from build123d import *

# Parameters (mm, degrees)
SZKIC1_R                    = 1.63
SZKIC1_R_2                  = 1.627886045
SZKIC1_R_3                  = 1.634186666
SZKIC1_R_4                  = 1.631321013
DODANIE_WYCI_GNI_CIE1_DEPTH = 37.7
SZKIC2_W                    = 96.882996132
SZKIC2_H                    = 10
WYTNIJ_WYCI_GNI_CIE1_DEPTH  = 3.027599165
SZKIC4_W                    = 27.7
SZKIC4_H                    = 3.027599165
DODANIE_WYCI_GNI_CIE2_DEPTH = 4.6
SZKIC5_W                    = 27.7
SZKIC5_H                    = 3.027593756
DODANIE_WYCI_GNI_CIE4_DEPTH = 4.6
WYTNIJ_WYCI_GNI_CIE2_REACH  = 74.407
SZKIC6_R                    = 2.5
SZKIC7_W                    = 110.003784397
SZKIC7_H                    = 59.74457964
WYTNIJ_WYCI_GNI_CIE4_DEPTH  = 30.7


with BuildPart() as part:
    # Szkic1 → Dodanie-wyciągnięcie1 (new body)
    with BuildSketch(Plane(origin=(0, 0, 0), x_dir=(-1, 0, 0), z_dir=(0, 0, 1))):
        with BuildLine():
            Line((-42.206476447, -1.143440143), (-42.187291437, -4.170973113))
            Line((-42.187291437, -4.170973113), (54.693759689, -3.557073712))
            Line((54.693759689, -3.557073712), (54.674575297, -0.529535329))
            Line((54.674575297, -0.529535329), (31.895047363, -0.673880775))
            ThreePointArc((31.895047363, -0.673880775), (30.123615765, 0.046208772), (29.379274421, 1.807587444))
            Line((29.379274421, 1.807587444), (29.351860706, 5.515732081))
            ThreePointArc((29.351860706, 5.515732081), (27.236675167, 10.484490063), (22.240808109, 12.534826154))
            Line((22.240808109, 12.534826154), (20.472861468, 12.523590896))
            ThreePointArc((20.472861468, 12.523590896), (19.415024557, 12.077529638), (18.982423849, 11.01411711))
            Line((18.982423849, 11.01411711), (18.989158593, 9.951213651))
            ThreePointArc((18.989158593, 9.951213651), (19.04575769, 9.79437408), (19.188385802, 9.708006664))
            Line((19.188385802, 9.708006664), (22.37305409, 9.047530924))
            Line((22.37305409, 9.047530924), (22.37305409, 7.841359432))
            Line((22.37305409, 7.841359432), (14.677855674, 7.841359432))
            ThreePointArc((14.677855674, 7.841359432), (4.517774256, 5.390280076), (-5.642307162, 7.841359432))
            Line((-5.642307162, 7.841359432), (-11.13863745, 7.841359432))
            ThreePointArc((-11.13863745, 7.841359432), (-11.344351569, 7.733421748), (-11.372431243, 7.502813045))
            Line((-11.372431243, 7.502813045), (-9.580573211, 2.77167383))
            Line((-9.580573211, 2.77167383), (-9.53660226, 2.594556029))
            ThreePointArc((-9.53660226, 2.594556029), (-10.047085724, 1.71578131), (-10.990723107, 2.09312315))
            Line((-10.990723107, 2.09312315), (-11.062286258, 2.28207519))
            Line((-11.062286258, 2.28207519), (-13.125087597, 7.728600603))
            ThreePointArc((-13.125087597, 7.728600603), (-13.0127689, 8.651035416), (-12.189912428, 9.082786152))
            Line((-12.189912428, 9.082786152), (-11.351176976, 9.082786152))
            ThreePointArc((-11.351176976, 9.082786152), (-11.174400281, 9.156009457), (-11.101176976, 9.332786152))
            Line((-11.101176976, 9.332786152), (-11.101176976, 9.341072815))
            ThreePointArc((-11.101176976, 9.341072815), (-11.158575506, 9.873705952), (-11.328135423, 10.381881202))
            Line((-11.328135423, 10.381881202), (-11.52139656, 10.803947934))
            ThreePointArc((-11.52139656, 10.803947934), (-11.948131465, 11.44871119), (-12.551468508, 11.932246866))
            Line((-12.551468508, 11.932246866), (-15.002316135, 13.336662904))
            ThreePointArc((-15.002316135, 13.336662904), (-15.916443983, 13.645833839), (-16.879567484, 13.585754641))
            Line((-16.879567484, 13.585754641), (-17.376357402, 13.455449083))
            ThreePointArc((-17.376357402, 13.455449083), (-19.591854135, 11.040960081), (-18.31207326, 8.024282466))
            Line((-18.31207326, 8.024282466), (-15.235252345, 4.594263276))
            ThreePointArc((-15.235252345, 4.594263276), (-14.894447251, 2.450948387), (-16.707962408, 1.258845372))
            Line((-16.707962408, 1.258845372), (-16.931951142, 1.257044798))
            ThreePointArc((-16.931951142, 1.257044798), (-17.929768207, 0.793667315), (-18.054097125, -0.299447458))
            ThreePointArc((-18.054097125, -0.299447458), (-18.09762478, -0.768632421), (-18.511820167, -0.993290758))
            Line((-18.511820167, -0.993290758), (-42.206476447, -1.143440143))
        make_face()
        with Locations(Location((21.198480742, 2.425447379, 0), (0, 0, 180))):
            Circle(SZKIC1_R, mode=Mode.SUBTRACT)
        with Locations(Location((-4.937145948, 2.427386246, 0), (0, 0, 180))):
            Circle(SZKIC1_R_2, mode=Mode.SUBTRACT)
        with Locations(Location((3.802928012, 2.422545785, 0), (0, 0, 180))):
            Circle(SZKIC1_R_3, mode=Mode.SUBTRACT)
        with Locations(Location((12.538480742, 2.425447379, 0), (0, 0, 180))):
            Circle(SZKIC1_R_4, mode=Mode.SUBTRACT)
    extrude(amount=DODANIE_WYCI_GNI_CIE1_DEPTH)

    # Szkic2 → Wytnij-wyciągnięcie1 (cut)
    with BuildSketch(Plane(origin=(-0.02473498, 3.903491109, 0), x_dir=(0.9999799241630359, 0.006336503048932176, 0), z_dir=(-0.006336503048932176, 0.9999799241630359, 0))):
        with Locations((-6.228624191, -32.7)):
            Rectangle(SZKIC2_W, SZKIC2_H)
    extrude(amount=-WYTNIJ_WYCI_GNI_CIE1_DEPTH, mode=Mode.SUBTRACT)

    # Szkic4 → Dodanie-wyciągnięcie2 (add)
    with BuildSketch(Plane(origin=(-54.669024709, -0.346417396, 0), x_dir=(0, 0, 1), z_dir=(-0.9999799241630359, -0.006336503048932243, 0))):
        with Locations((13.85, 2.389769894)):
            Rectangle(SZKIC4_W, SZKIC4_H)
    extrude(amount=DODANIE_WYCI_GNI_CIE2_DEPTH)

    # Szkic5 → Dodanie-wyciągnięcie4 (add)
    with BuildSketch(Plane(origin=(42.212027201, 0.26749111, 0), x_dir=(0, 0, -1), z_dir=(0.9999799227968423, 0.00633671864778665, 0))):
        with Locations((-13.85, 2.389763497)):
            Rectangle(SZKIC5_W, SZKIC5_H)
    extrude(amount=DODANIE_WYCI_GNI_CIE4_DEPTH)

    # Wytnij-wyciągnięcie2: up to this face of the body (flat: up to its plane)
    wytnij_wyci_gni_cie2_end = Plane(part.part.faces().sort_by_distance((-45.584765156, 0.587134095, 13.85))[0])
    # Szkic6 → Wytnij-wyciągnięcie2 (cut, up to the picked face)
    with BuildSketch(Plane(origin=(-0.02473498, 3.903491109, 0), x_dir=(0.9999799241630359, 0.006336503048932172, 0), z_dir=(-0.006336503048932172, 0.9999799241630359, 0)), mode=Mode.PRIVATE) as wytnij_wyci_gni_cie2_sk1:
        with Locations((-53.770122257, -7.5)):
            Circle(SZKIC6_R)
    wytnij_wyci_gni_cie2_tool1 = split(extrude(wytnij_wyci_gni_cie2_sk1.sketch, amount=-WYTNIJ_WYCI_GNI_CIE2_REACH, mode=Mode.PRIVATE), bisect_by=wytnij_wyci_gni_cie2_end, keep=Keep.BOTH, mode=Mode.PRIVATE)
    # Szkic6 → Wytnij-wyciągnięcie2 (cut, up to the picked face)
    with BuildSketch(Plane(origin=(-0.02473498, 3.903491109, 0), x_dir=(0.9999799241630359, 0.006336503048932172, 0), z_dir=(-0.006336503048932172, 0.9999799241630359, 0)), mode=Mode.PRIVATE) as wytnij_wyci_gni_cie2_sk2:
        with Locations((41.312873875, -7.5)):
            Circle(SZKIC6_R)
    wytnij_wyci_gni_cie2_tool2 = split(extrude(wytnij_wyci_gni_cie2_sk2.sketch, amount=-WYTNIJ_WYCI_GNI_CIE2_REACH, mode=Mode.PRIVATE), bisect_by=wytnij_wyci_gni_cie2_end, keep=Keep.BOTH, mode=Mode.PRIVATE)
    add(wytnij_wyci_gni_cie2_tool1.solids().sort_by(Axis((-53.793778, 3.562777, 7.5), (0.006336503048932172, -0.9999799241630359, 0)))[0], mode=Mode.SUBTRACT)
    add(wytnij_wyci_gni_cie2_tool2.solids().sort_by(Axis((41.28731, 4.16527, 7.5), (0.006336503048932172, -0.9999799241630359, 0)))[0], mode=Mode.SUBTRACT)

    # Szkic7 → Wytnij-wyciągnięcie4 (cut)
    with BuildSketch(Plane(origin=(0, 0, 0), x_dir=(-1, 0, 0), z_dir=(0, 0, -1))):
        with Locations((7.955893791, -24.915165787)):
            Rectangle(SZKIC7_W, SZKIC7_H)
    extrude(amount=-WYTNIJ_WYCI_GNI_CIE4_DEPTH, mode=Mode.SUBTRACT)


with BuildPart() as wytnij_wyci_gni_cie4_kept_piece:
    # of the separate pieces the step leaves, the one the design keeps (wytnij_wyci_gni_cie4_pieces_kept)
    add(part.part.solids().sort_by_distance((18.31207326, -8.024282466, 30.7))[0])


solid = wytnij_wyci_gni_cie4_kept_piece.part
Check sheet for the modelled part. Datum: model origin and axes. Units: mm. A direction names the side the tool comes from. Give positions to 0.01 mm unless a question says otherwise; leave off trailing zeros. Write each loop counter-clockwise with the first axis right and the second up, starting at its lowest first coordinate (ties: lowest second). Pieces come first, ordered by that corner, then holes. Notation, with made-up numbers: (41, -36.5) -> (65, -36.5) arc R31 ccw to (65, -11.5) -> close; hole circle Ø10 at (-27.75, 80). An arc over 180 degrees is marked (long way). Use one line per item in the form item = value. Start each with the question number.
1. Section check A-A (x = 5). Record the cut outline in (y, z).
2. Go/stop test with flat-tipped pins: P1, Ø3, axis at x = -18.5, z = 34, coming from the +Y side; P2, Ø1.6, axis at x = 7.5, z = 35, coming from the -Y side; P3, Ø1.3, axis at y = -8, z = 32.5, coming from the +X side; P4, Ø2.5, axis at x = -12.54, y = -2.43, coming from the +Z side. Record where each tip stops, or that it passes through.
3. Section check B-B (y = -6.5). Record the cut outline in (x, z).
4. Mould release check, pull along Y, two halves, no side actions. Record for faces 5 (the cylindrical face through (17.92, -0.81, 34.15)), 6 (the flat face through (-6, -5, 30.7)), 7 (the flat face through (12, -9.083, 34)), 8 (the flat face through (13.76, -12.625, 34.151)): pulls with the +Y half, pulls with the -Y half, needs draft (parallel to the pull), parting line crosses it, or undercut.
5. Section check D-D (x = -12). Record the cut outline in (y, z).
6. Thickness scan on line 1 along X through (y, z) = (-7.75, 37); line 2 along X through (y, z) = (-7.25, 34.5); line 3 along X through (y, z) = (-2.5, 34). Record the ranges inside material, lowest first. Write a range as from..to.
7. Section check C-C (y = -3.5). Record the cut outline in (x, z), and give its area (3 significant figures).
8. Access from +Z, -Z, +X, -X, +Y, -Y to the whole of each face (thin tool, end or side, straight path). Record for faces 1 (the flat face through (-22.373, -8, 34)), 2 (the flat face through (16.795, -6.333, 34.151)), 3 (the flat face through (-6, -5, 37.7)), 4 (the cylindrical face through (11.157, -9.866, 34.151)).
Conclusion:
q1.outline = (-7.53, 30.7) -> (-4.05, 30.7) -> (-4.05, 37.7) -> (-7.53, 37.7) -> close; (-0.8, 30.7) -> (0.91, 30.7) -> (0.91, 37.7) -> (-0.8, 37.7) -> close
q2.P1 = 0.77
q2.P2 = -7.84
q2.P3 = 18.98
q2.P4 = through
q3.outline = (-29.27, 30.7) -> (-11.46, 30.7) -> (-11.46, 37.7) -> (-29.27, 37.7) -> close; (2.43, 30.7) -> (10.99, 30.7) -> (10.99, 37.7) -> (2.43, 37.7) -> close; (12.66, 30.7) -> (16.94, 30.7) -> (16.94, 37.7) -> (12.66, 37.7) -> close
q4.face_5 = undercut
q4.face_6 = needs draft
q4.face_7 = undercut
q4.face_8 = pulls with the -Y half
q5.outline = (-6.68, 30.7) -> (-3.97, 30.7) -> (-3.97, 37.7) -> (-6.68, 37.7) -> close; (-0.89, 30.7) -> (0.8, 30.7) -> (0.8, 37.7) -> (-0.89, 37.7) -> close
q6.line_1 = -28.96..-14.5, 5.46..11.33, 13.13..18.07
q6.line_2 = -29.11..-13.43, 4.39..11.28, 12.94..17.62
q6.line_3 = -29.37..-22.83, -19.57..-14.17, -10.91..-5.44, -2.17..3.31, 6.56..9.52, 11.14..14.87
q7.outline = (-29.37, 30.7) -> (-22.42, 30.7) -> (-22.42, 37.7) -> (-29.37, 37.7) -> close; (-19.97, 30.7) -> (-13.77, 30.7) -> (-13.77, 37.7) -> (-19.97, 37.7) -> close; (-11.31, 30.7) -> (-5.03, 30.7) -> (-5.03, 37.7) -> (-11.31, 37.7) -> close; (-2.57, 30.7) -> (3.71, 30.7) -> (3.71, 37.7) -> (-2.57, 37.7) -> close; (6.16, 30.7) -> (9.86, 30.7) -> (9.86, 37.7) -> (6.16, 37.7) -> close; (11.52, 30.7) -> (14.74, 30.7) -> (14.74, 37.7) -> (11.52, 37.7) -> close
q7.area = 228 mm²
q8.face_1 = +Z, -Z
q8.face_2 = +Z, -Z, +X
q8.face_3 = +Z, +X, -X, +Y, -Y
q8.face_4 = +Z, -Z, -Y
